Model file for the job. Use its own axes, mm. A direction names the side the tool comes from. Round coordinates to 2 decimals unless told otherwise and drop trailing zeros. Order: outer loops, then holes, each group sorted by start corner. A loop starts at its lowest first (then second) coordinate and runs counter-clockwise, first axis right, second up. Notation, with made-up numbers: (-28, 4) -> (20, 4) arc R35 ccw to (20, 37) -> close; hole circle Ø1 at (32.5, 4). An arc over 180 degrees is marked (long way). Answer as CSV lines item,"result".
```python
from build123d import *

# Parameters (mm, degrees)
AUFSATZ_LINEAR_AUSTRAGEN1_DEPTH = 10
SKIZZE2_R                       = 1.75
SCHNITT_LINEAR_AUSTRAGEN1_DEPTH = 62.985320843
SKIZZE4_R                       = 2.2
SCHNITT_LINEAR_AUSTRAGEN3_DEPTH = 73.202839279
VERRUNDUNG1_R                   = 10


with BuildPart() as part:
    # Skizze1 → Aufsatz-Linear austragen1 (new body)
    with BuildSketch(Plane.XY):
        with BuildLine():
            Line((0.5, -26.695317942), (0.5, -30.695928069))
            Line((0.5, -30.695928069), (0.5, -36.695928069))
            Line((0.5, -36.695928069), (2, -36.695928069))
            Line((2, -36.695928069), (2, -30.634784151))
            ThreePointArc((2, -30.634784151), (29.374903671, -8.922165338), (18.7, 24.34748447))
            Line((18.7, 24.34748447), (18.7, 51.7))
            Line((18.7, 51.7), (10.2, 51.7))
            Line((10.2, 51.7), (10.2, 31.7))
            Line((10.2, 31.7), (-10.2, 31.7))
            Line((-10.2, 31.7), (-10.2, 51.7))
            Line((-10.2, 51.7), (-18.7, 51.7))
            Line((-18.7, 51.7), (-18.7, 24.34748447))
            ThreePointArc((-18.7, 24.34748447), (-29.374903671, -8.922165338), (-2, -30.634784151))
            Line((-2, -30.634784151), (-2, -36.695928069))
            Line((-2, -36.695928069), (-0.5, -36.695928069))
            Line((-0.5, -36.695928069), (-0.5, -30.695928069))
            Line((-0.5, -30.695928069), (-0.5, -26.695317942))
            ThreePointArc((-0.5, -26.695317942), (0, 26.7), (0.5, -26.695317942))
        make_face()
    extrude(amount=AUFSATZ_LINEAR_AUSTRAGEN1_DEPTH)

    # Skizze2 → Schnitt-Linear austragen1 (cut, through all)
    with BuildSketch(Plane.ZY.offset(2)):
        with Locations(Location((5, -33.66535611, 0), (0, 0, 90))):
            Circle(SKIZZE2_R)
    extrude(amount=-SCHNITT_LINEAR_AUSTRAGEN1_DEPTH, mode=Mode.SUBTRACT)

    # Skizze4 → Schnitt-Linear austragen3 (cut, through all)
    with BuildSketch(Plane.ZY.offset(18.7)):
        with Locations(Location((5, 41.7, 0), (0, 0, 270))):
            Circle(SKIZZE4_R)
    extrude(amount=-SCHNITT_LINEAR_AUSTRAGEN3_DEPTH, mode=Mode.SUBTRACT)

    # Verrundung1
    verrundung1_edges = [part.edges().sort_by_distance(p)[0] for p in [
        (-18.7, 24.34748447, 5),
        (18.7, 24.34748447, 5),
    ]]
    fillet(verrundung1_edges, radius=VERRUNDUNG1_R)


solid = part.part
```
Q1. Mould opens along Z. For faces 1 (the cylindrical face through (1.24, -35.414, 4.923)), 2 (the flat face through (0, 27, 10)), 3 (the flat face through (-10.2, 39, 5)) say: +Z half, -Z half, draft (parallel to the pull), parting line (faces both ways), or undercut.
Checks:
face 1,"undercut"
face 2,"+Z half"
face 3,"draft"
Q2. Saw through at B-B (x = -12). Write the cut outline in (y, z), plus the area to 3 significant figures.
Checks:
outline,"(-28.26, 0) -> (-23.85, 0) -> (-23.85, 10) -> (-28.26, 10) -> close; (23.85, 0) -> (51.7, 0) -> (51.7, 10) -> (23.85, 10) -> close; hole circle Ø4.4 at (41.7, 5)"
area,"307 mm²"
Q3. Tool access for faces 4 (the flat face through (-2, -32, 4)), 5 (the flat face through (10.2, 44.1, 4.9)), 6 (the flat face through (-0.5, -31.766, 4.93)), 7 (the flat face through (18.7, 40, 3)), 8 (the flat face through (2, -32, 4)): list every direction of +Z, -Z, +X, -X, +Y, -Y with a clear straight run to the whole face (end or side of a thin tool).
Checks:
face 4,"+Z, -Z, -X, -Y"
face 5,"+Z, -Z, +Y"
face 6,"+Z, -Z, -Y"
face 7,"+Z, -Z, +X, +Y"
face 8,"+Z, -Z, +X, -Y"
Q4. Saw through at D-D (z = 1.75). Write the cut outline in (x, y).
Checks:
outline,"(-21.65, 21.77) arc R30.7 ccw to (-2, -30.63) -> (-2, -36.7) -> (-0.5, -36.7) -> (-0.5, -26.7) arc R26.7 cw (long way) to (0.5, -26.7) -> (0.5, -36.7) -> (2, -36.7) -> (2, -30.63) arc R30.7 ccw to (21.65, 21.77) arc R10 cw to (18.7, 28.86) -> (18.7, 51.7) -> (10.2, 51.7) -> (10.2, 31.7) -> (-10.2, 31.7) -> (-10.2, 51.7) -> (-18.7, 51.7) -> (-18.7, 28.86) arc R10 cw to start"
Q5. Saw through at C-C (y = 0). Write the cut outline in (x, z), plus the area to 3 significant figures.
Checks:
outline,"(-30.7, 0) -> (-26.7, 0) -> (-26.7, 10) -> (-30.7, 10) -> close; (26.7, 0) -> (30.7, 0) -> (30.7, 10) -> (26.7, 10) -> close"
area,"80.0 mm²"
Q6. Saw through at A-A (y = 41.7). Write the cut outline in (x, z), plus the area to 3 significant figures.
Checks:
outline,"(-18.7, 0) -> (-10.2, 0) -> (-10.2, 2.8) -> (-18.7, 2.8) -> close; (-18.7, 7.2) -> (-10.2, 7.2) -> (-10.2, 10) -> (-18.7, 10) -> close; (10.2, 0) -> (18.7, 0) -> (18.7, 2.8) -> (10.2, 2.8) -> close; (10.2, 7.2) -> (18.7, 7.2) -> (18.7, 10) -> (10.2, 10) -> close"
area,"95.2 mm²"
Q7. Flat gauge pins, fed straight in: pin 1 (3 mm diameter, centred on x = -4.5, z = 4, fed in from +Y); pin 2 (2 mm diameter, centred on y = -33.67, z = 5, fed in from +X); pin 3 (1 mm diameter, centred on y = -12.5, z = 6.5, fed in from +X); pin 4 (5.5 mm diameter, centred on y = 41.7, z = 5, fed in from +X). Where does each tip first touch, or does it go through?
Checks:
pin 1,"y = 31.7"
pin 2,"through"
pin 3,"x = 28.26"
pin 4,"x = 18.7"
Q8. Wall check: L1, parallel to Z at x = -11.75, y = 41.7; L2, parallel to Y at x = 1.3, z = 5; L3, parallel to X at y = 37.5, z = 7.25. Give the ranges that are in metal, low to high. Write a range as [from, to].
Checks:
L1,"[0, 2.8], [7.2, 10]"
L2,"[-36.7, -35.42], [-31.92, -26.67], [26.67, 31.7]"
L3,"[-18.7, -10.2], [10.2, 18.7]"
